```python
from build123d import *

# Parameters (mm, degrees)
CYLINDER135_R          = 1.8
CYLINDER135_DEPTH      = 34
CYLINDER135_ROLL_ANGLE = 90
CYLINDER134_R          = 1.8
CYLINDER134_DEPTH      = 34
CYLINDER134_ROLL_ANGLE = 90
CYLINDER137_R          = 3
CYLINDER137_DEPTH      = 34
CYLINDER137_ROLL_ANGLE = 90
CYLINDER136_R          = 3
CYLINDER136_DEPTH      = 34
CYLINDER136_ROLL_ANGLE = 90
CYLINDER123_R          = 1.8
CYLINDER123_DEPTH      = 34
CYLINDER123_ROLL_ANGLE = 90
CYLINDER122_R          = 1.8
CYLINDER122_DEPTH      = 34
CYLINDER122_ROLL_ANGLE = 90
CYLINDER125_R          = 1.8
CYLINDER125_DEPTH      = 34
CYLINDER125_ROLL_ANGLE = 90
CYLINDER124_R          = 1.8
CYLINDER124_DEPTH      = 34
CYLINDER124_ROLL_ANGLE = 90
CYLINDER127_R          = 3
CYLINDER127_DEPTH      = 34
CYLINDER127_ROLL_ANGLE = 90
CYLINDER126_R          = 3
CYLINDER126_DEPTH      = 34
CYLINDER126_ROLL_ANGLE = 90
CYLINDER129_R          = 3
CYLINDER129_DEPTH      = 34
CYLINDER129_ROLL_ANGLE = 90
CYLINDER128_R          = 3
CYLINDER128_DEPTH      = 34
CYLINDER128_ROLL_ANGLE = 90
CYLINDER131_R          = 1.8
CYLINDER131_DEPTH      = 34
CYLINDER131_ROLL_ANGLE = 90
CYLINDER130_R          = 1.8
CYLINDER130_DEPTH      = 34
CYLINDER130_ROLL_ANGLE = 90
CYLINDER133_R          = 1.8
CYLINDER133_DEPTH      = 34
CYLINDER133_ROLL_ANGLE = 90
CYLINDER132_R          = 1.8
CYLINDER132_DEPTH      = 34
CYLINDER132_ROLL_ANGLE = 90
BOX061_W               = 50
BOX061_H               = 6
BOX061_DEPTH           = 67
FILLET055_R            = 6


with BuildPart() as cilindro089:
    # Cylinder135 → Cylinder135 (new body)
    with BuildSketch(Plane.XY):
        Circle(CYLINDER135_R)
    extrude(amount=CYLINDER135_DEPTH)


with BuildPart() as cilindro089_1:
    # Cylinder135 roll: moved
    add(cilindro089.part.rotate(Axis((0, 0, 0), (1, 0, 0)), CYLINDER135_ROLL_ANGLE))


with BuildPart() as cilindro089_2:
    # Cylinder135 placement: moved
    add(cilindro089_1.part.moved(Location((24, -10, 64))))


with BuildPart() as fusion079:
    # Cylinder134 → Cylinder134 (new body)
    with BuildSketch(Plane.XY):
        Circle(CYLINDER134_R)
    extrude(amount=CYLINDER134_DEPTH)


with BuildPart() as fusion079_1:
    # Cylinder134 roll: moved
    add(fusion079.part.rotate(Axis((0, 0, 0), (1, 0, 0)), CYLINDER134_ROLL_ANGLE))


with BuildPart() as fusion079_2:
    # Cylinder134 placement: moved
    add(fusion079_1.part.moved(Location((40, -10, 64))))

    # Fusion079: union Cilindro089
    add(cilindro089_2.part)


with BuildPart() as fusion079_3:
    # Fusion079 placement: moved
    add(fusion079_2.part.moved(Location((0, 0, -8))))


with BuildPart() as cilindro091:
    # Cylinder137 → Cylinder137 (new body)
    with BuildSketch(Plane.XY):
        Circle(CYLINDER137_R)
    extrude(amount=CYLINDER137_DEPTH)


with BuildPart() as cilindro091_1:
    # Cylinder137 roll: moved
    add(cilindro091.part.rotate(Axis((0, 0, 0), (1, 0, 0)), CYLINDER137_ROLL_ANGLE))


with BuildPart() as cilindro091_2:
    # Cylinder137 placement: moved
    add(cilindro091_1.part.moved(Location((24, -10, 64))))


with BuildPart() as fusion080:
    # Cylinder136 → Cylinder136 (new body)
    with BuildSketch(Plane.XY):
        Circle(CYLINDER136_R)
    extrude(amount=CYLINDER136_DEPTH)


with BuildPart() as fusion080_1:
    # Cylinder136 roll: moved
    add(fusion080.part.rotate(Axis((0, 0, 0), (1, 0, 0)), CYLINDER136_ROLL_ANGLE))


with BuildPart() as fusion080_2:
    # Cylinder136 placement: moved
    add(fusion080_1.part.moved(Location((40, -10, 64))))

    # Fusion080: union Cilindro091
    add(cilindro091_2.part)


with BuildPart() as fusion080_3:
    # Fusion080 placement: moved
    add(fusion080_2.part.moved(Location((0, 23, -8))))


with BuildPart() as cilindro077:
    # Cylinder123 → Cylinder123 (new body)
    with BuildSketch(Plane.XY):
        Circle(CYLINDER123_R)
    extrude(amount=CYLINDER123_DEPTH)


with BuildPart() as cilindro077_1:
    # Cylinder123 roll: moved
    add(cilindro077.part.rotate(Axis((0, 0, 0), (1, 0, 0)), CYLINDER123_ROLL_ANGLE))


with BuildPart() as cilindro077_2:
    # Cylinder123 placement: moved
    add(cilindro077_1.part.moved(Location((24, -10, 64))))


with BuildPart() as fusion070:
    # Cylinder122 → Cylinder122 (new body)
    with BuildSketch(Plane.XY):
        Circle(CYLINDER122_R)
    extrude(amount=CYLINDER122_DEPTH)


with BuildPart() as fusion070_1:
    # Cylinder122 roll: moved
    add(fusion070.part.rotate(Axis((0, 0, 0), (1, 0, 0)), CYLINDER122_ROLL_ANGLE))


with BuildPart() as fusion070_2:
    # Cylinder122 placement: moved
    add(fusion070_1.part.moved(Location((40, -10, 64))))

    # Fusion070: union Cilindro077
    add(cilindro077_2.part)


with BuildPart() as fusion070_3:
    # Fusion070 placement: moved
    add(fusion070_2.part.moved(Location((0, 0, -8))))


with BuildPart() as cilindro079:
    # Cylinder125 → Cylinder125 (new body)
    with BuildSketch(Plane.XY):
        Circle(CYLINDER125_R)
    extrude(amount=CYLINDER125_DEPTH)


with BuildPart() as cilindro079_1:
    # Cylinder125 roll: moved
    add(cilindro079.part.rotate(Axis((0, 0, 0), (1, 0, 0)), CYLINDER125_ROLL_ANGLE))


with BuildPart() as cilindro079_2:
    # Cylinder125 placement: moved
    add(cilindro079_1.part.moved(Location((24, -10, 61))))


with BuildPart() as fusion072:
    # Cylinder124 → Cylinder124 (new body)
    with BuildSketch(Plane.XY):
        Circle(CYLINDER124_R)
    extrude(amount=CYLINDER124_DEPTH)


with BuildPart() as fusion072_1:
    # Cylinder124 roll: moved
    add(fusion072.part.rotate(Axis((0, 0, 0), (1, 0, 0)), CYLINDER124_ROLL_ANGLE))


with BuildPart() as fusion072_2:
    # Cylinder124 placement: moved
    add(fusion072_1.part.moved(Location((40, -10, 61))))

    # Fusion071: union Cilindro079
    add(cilindro079_2.part)


with BuildPart() as fusion072_3:
    # Fusion071 placement: moved
    add(fusion072_2.part.moved(Location((0, 0, 35))))

    # Fusion072: union Fusion070
    add(fusion070_3.part)


with BuildPart() as cilindro081:
    # Cylinder127 → Cylinder127 (new body)
    with BuildSketch(Plane.XY):
        Circle(CYLINDER127_R)
    extrude(amount=CYLINDER127_DEPTH)


with BuildPart() as cilindro081_1:
    # Cylinder127 roll: moved
    add(cilindro081.part.rotate(Axis((0, 0, 0), (1, 0, 0)), CYLINDER127_ROLL_ANGLE))


with BuildPart() as cilindro081_2:
    # Cylinder127 placement: moved
    add(cilindro081_1.part.moved(Location((24, -10, 64))))


with BuildPart() as fusion073:
    # Cylinder126 → Cylinder126 (new body)
    with BuildSketch(Plane.XY):
        Circle(CYLINDER126_R)
    extrude(amount=CYLINDER126_DEPTH)


with BuildPart() as fusion073_1:
    # Cylinder126 roll: moved
    add(fusion073.part.rotate(Axis((0, 0, 0), (1, 0, 0)), CYLINDER126_ROLL_ANGLE))


with BuildPart() as fusion073_2:
    # Cylinder126 placement: moved
    add(fusion073_1.part.moved(Location((40, -10, 64))))

    # Fusion073: union Cilindro081
    add(cilindro081_2.part)


with BuildPart() as cilindro083:
    # Cylinder129 → Cylinder129 (new body)
    with BuildSketch(Plane.XY):
        Circle(CYLINDER129_R)
    extrude(amount=CYLINDER129_DEPTH)


with BuildPart() as cilindro083_1:
    # Cylinder129 roll: moved
    add(cilindro083.part.rotate(Axis((0, 0, 0), (1, 0, 0)), CYLINDER129_ROLL_ANGLE))


with BuildPart() as cilindro083_2:
    # Cylinder129 placement: moved
    add(cilindro083_1.part.moved(Location((24, -10, 61))))


with BuildPart() as fusion075:
    # Cylinder128 → Cylinder128 (new body)
    with BuildSketch(Plane.XY):
        Circle(CYLINDER128_R)
    extrude(amount=CYLINDER128_DEPTH)


with BuildPart() as fusion075_1:
    # Cylinder128 roll: moved
    add(fusion075.part.rotate(Axis((0, 0, 0), (1, 0, 0)), CYLINDER128_ROLL_ANGLE))


with BuildPart() as fusion075_2:
    # Cylinder128 placement: moved
    add(fusion075_1.part.moved(Location((40, -10, 61))))

    # Fusion074: union Cilindro083
    add(cilindro083_2.part)


with BuildPart() as fusion075_3:
    # Fusion074 placement: moved
    add(fusion075_2.part.moved(Location((0, 0, 35))))

    # Fusion075: union Fusion073
    add(fusion073_2.part)


with BuildPart() as fusion075_4:
    # Fusion075 placement: moved
    add(fusion075_3.part.moved(Location((0, 25, 0))))


with BuildPart() as cilindro085:
    # Cylinder131 → Cylinder131 (new body)
    with BuildSketch(Plane.XY):
        Circle(CYLINDER131_R)
    extrude(amount=CYLINDER131_DEPTH)


with BuildPart() as cilindro085_1:
    # Cylinder131 roll: moved
    add(cilindro085.part.rotate(Axis((0, 0, 0), (1, 0, 0)), CYLINDER131_ROLL_ANGLE))


with BuildPart() as cilindro085_2:
    # Cylinder131 placement: moved
    add(cilindro085_1.part.moved(Location((16, -10, 63))))


with BuildPart() as fusion076:
    # Cylinder130 → Cylinder130 (new body)
    with BuildSketch(Plane.XY):
        Circle(CYLINDER130_R)
    extrude(amount=CYLINDER130_DEPTH)


with BuildPart() as fusion076_1:
    # Cylinder130 roll: moved
    add(fusion076.part.rotate(Axis((0, 0, 0), (1, 0, 0)), CYLINDER130_ROLL_ANGLE))


with BuildPart() as fusion076_2:
    # Cylinder130 placement: moved
    add(fusion076_1.part.moved(Location((50, -10, 63))))

    # Fusion076: union Cilindro085
    add(cilindro085_2.part)


with BuildPart() as cilindro087:
    # Cylinder133 → Cylinder133 (new body)
    with BuildSketch(Plane.XY):
        Circle(CYLINDER133_R)
    extrude(amount=CYLINDER133_DEPTH)


with BuildPart() as cilindro087_1:
    # Cylinder133 roll: moved
    add(cilindro087.part.rotate(Axis((0, 0, 0), (1, 0, 0)), CYLINDER133_ROLL_ANGLE))


with BuildPart() as cilindro087_2:
    # Cylinder133 placement: moved
    add(cilindro087_1.part.moved(Location((16, -10, 63))))


with BuildPart() as fusion078:
    # Cylinder132 → Cylinder132 (new body)
    with BuildSketch(Plane.XY):
        Circle(CYLINDER132_R)
    extrude(amount=CYLINDER132_DEPTH)


with BuildPart() as fusion078_1:
    # Cylinder132 roll: moved
    add(fusion078.part.rotate(Axis((0, 0, 0), (1, 0, 0)), CYLINDER132_ROLL_ANGLE))


with BuildPart() as fusion078_2:
    # Cylinder132 placement: moved
    add(fusion078_1.part.moved(Location((50, -10, 63))))

    # Fusion077: union Cilindro087
    add(cilindro087_2.part)


with BuildPart() as fusion078_3:
    # Fusion077 placement: moved
    add(fusion078_2.part.moved(Location((0, 0, 43))))

    # Fusion078: union Fusion076
    add(fusion076_2.part)


with BuildPart() as fillet055:
    # Box061 → Box061 (new body)
    with BuildSketch(Plane(origin=(8, -23, 49), x_dir=(1, 0, 0), z_dir=(0, 0, 1))):
        with Locations((25, 3)):
            Rectangle(BOX061_W, BOX061_H)
    extrude(amount=BOX061_DEPTH)

    # Cut140: cut Fusion078
    add(fusion078_3.part, mode=Mode.SUBTRACT)

    # Cut141: cut Fusion075
    add(fusion075_4.part, mode=Mode.SUBTRACT)

    # Cut142: cut Fusion072
    add(fusion072_3.part, mode=Mode.SUBTRACT)

    # Cut143: cut Fusion080
    add(fusion080_3.part, mode=Mode.SUBTRACT)

    # Cut144: cut Fusion079
    add(fusion079_3.part, mode=Mode.SUBTRACT)

    # Fillet055
    fillet055_edges = [fillet055.edges().sort_by_distance(p)[0] for p in [
        (8, -20, 116),
        (8, -20, 49),
        (58, -20, 116),
        (58, -20, 49),
    ]]
    fillet(fillet055_edges, radius=FILLET055_R)


solid = fillet055.part
```
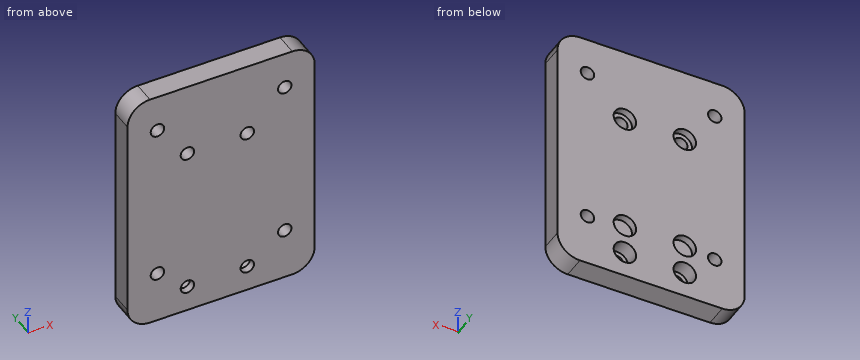
Model file for the job. Use its own axes, mm. Round coordinates to 2 decimals unless told otherwise and drop trailing zeros. Order: outer loops, then holes, each group sorted by start corner. A loop starts at its lowest first (then second) coordinate and runs counter-clockwise, first axis right, second up. Notation, with made-up numbers: (-17.5, -27.75) -> (-6.5, -27.75) arc R10 ccw to (-6.5, -9.75) -> close; hole circle Ø2 at (-6.5, 60). An arc over 180 degrees is marked (long way). Use one line per item in the form item = value.
Item 1: Cut at D-D, the plane z = 106. Write the cut outline in (x, y).
Returned:
outline = (8, -23) -> (14.2, -23) -> (14.2, -17) -> (8, -17) -> close; (17.8, -23) -> (48.2, -23) -> (48.2, -17) -> (17.8, -17) -> close; (51.8, -23) -> (58, -23) -> (58, -17) -> (51.8, -17) -> close
Item 2: Flat gauge pins, fed straight in: pin 1 Ø1.8 at (x, z) = (23.5, 63.5) entering from +Y; pin 2 Ø3 at (x, z) = (24, 96) entering from -Y. Where does each tip first touch, or does it go through?
Returned:
pin_1 = -19
pin_2 = through
Item 3: Cut at B-B, the plane x = 50. Write the cut outline in (y, z).
Returned:
outline = (-23, 49) -> (-17, 49) -> (-17, 61.2) -> (-23, 61.2) -> close; (-23, 64.8) -> (-17, 64.8) -> (-17, 104.2) -> (-23, 104.2) -> close; (-23, 107.8) -> (-17, 107.8) -> (-17, 116) -> (-23, 116) -> close
Item 4: Drill centre lines: line 1 (Z direction, x = 24, y = -19.3); line 2 (Z direction, x = 16, y = -19.4); line 3 (Z direction, x = 24, y = -17.3). Where is each one in solid material? Low to high.
Returned:
line_1 = 49 to 53, 59 to 94.2, 97.8 to 116
line_2 = 49 to 61.2, 64.8 to 104.2, 107.8 to 116
line_3 = 49 to 53, 59 to 61, 67 to 93, 99 to 116
Item 5: Cut at C-C, the plane y = -18.15. Give the number of separate pieces and of enclosed holes in the cut face, and give its area (3 significant figures).
Returned:
separate_pieces = 1
enclosed_holes = 10
area = 3,110 mm^2
Item 6: Cut at A-A, the plane z = 96. Write the cut outline in (x, y), and give its area (3 significant figures).
Returned:
outline = (8, -23) -> (22.2, -23) -> (22.2, -19) -> (21, -19) -> (21, -17) -> (8, -17) -> close; (25.8, -23) -> (38.2, -23) -> (38.2, -19) -> (37, -19) -> (37, -17) -> (27, -17) -> (27, -19) -> (25.8, -19) -> close; (41.8, -23) -> (58, -23) -> (58, -17) -> (43, -17) -> (43, -19) -> (41.8, -19) -> close
area = 247 mm^2
